Read the model definition and answer for the solid it produces. Units are mm, in the model's axes. Face numbers are marked on the shaded views. A direction names the side the tool comes from. Coordinates: 2 decimals unless noted, no trailing zeros. Loops run counter-clockwise (first coordinate to the right, second up) from the corner with the lowest first, then second, coordinate; pieces in that order, holes last. Notation, with made-up numbers: M 75,5 L 112,5 A24 ccw 112,27 Z; hole C 73,47.25 d5. An arc over 180 degrees is marked long. One line per item, written item: value. Start each with the question number.
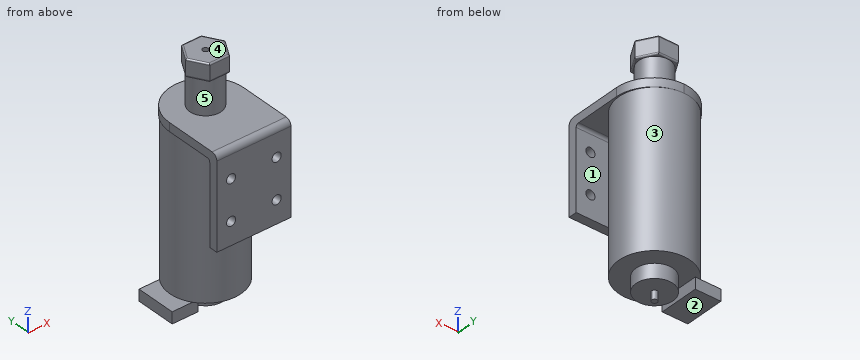
Autodesk Inventor part; units mm, degrees
ref_plane "YZ Plane" through (0, 0, 0) normal (1, 0, 0) x (0, 1, 0)
ref_plane "XZ Plane" through (0, 0, 0) normal (0, 1, 0) x (-1, 0, 0)
ref_plane "XY Plane" through (0, 0, 0) normal (0, 0, 1) x (1, 0, 0)
sketch "Эскиз1" plane through (0, 0, 0) normal (0, 1, 0) x (-1, 0, 0)
  line L0 (0, 0) -> (-26, 0)
  line L1 (0, -32) -> (-26, -32)
  line L2 (-26, -32) -> (0, -32)
  line L3 (0, -32) -> (0, 0)
  line L4 (0, 0) -> (-26, 0)
  line L5 (-26, 0) -> (-26, -32)
extrude "Выдавливание1" add sketch "Эскиз1" along normal blind 3
sketch "Эскиз2" plane through (0, 3, 0) normal (0, 1, 0) x (1, 0, 0)
  line L0 (0, 0) -> (26, 0)
  line L1 (26, 0) -> (26, 33)
  line L2 (0, 0) -> (26, 0)
  line L3 (26, 0) -> (26, 3)
  line L4 (26, 3) -> (0, 3)
  line L5 (0, 3) -> (0, 0)
  dimension "d4" = 3
extrude "Выдавливание2" add sketch "Эскиз2" along normal blind 30
sketch "Эскиз3" plane through (26, 3, -3) normal (0, 0, -1) x (-1, 0, 0)
  line L0 (0, 0) -> (26, 0)
  line L1 (13, 0) -> (13, 5)
  line L2 (13, 5) -> (13, 17.5)
  circle A0 centre (13, 17.5) radius 12.5
  point P0 (26, -3)
  dimension "d7" = 5
  dimension "d8" = 12.5
extrude "Выдавливание3" add sketch "Эскиз3" along normal blind 61.8
sketch "Эскиз4" plane through (13, 20.5, -64.8) normal (0, 0, -1) x (-1, 0, 0)
  circle A0 centre (0, 0) radius 6.5
  circle A1 centre (0, 0) radius 12.5
  point P0 (13, -20.5)
  dimension "d11" = 13
extrude "Выдавливание4" cut sketch "Эскиз4" against normal blind 8
sketch "Эскиз5" plane through (13, 20.5, -64.8) normal (0, 0, -1) x (-1, 0, 0)
  circle A0 centre (0, 0) radius 1
  circle A1 centre (0, 0) radius 6.5
  point P0 (13, -20.5)
  dimension "d14" = 2
extrude "Выдавливание5" cut sketch "Эскиз5" against normal blind 3
sketch "Эскиз6" plane through (13, 20.5, -56.8) normal (0, 0, -1) x (-1, 0, 0)
  circle A0 centre (0, 0) radius 12.5
  line L0 (-12.5, 0) -> (8.5, 0)
  line L1 (8.5, 0) -> (8.5, 7)
  line L2 (8.5, 7) -> (17.5, 7)
  line L3 (17.5, 7) -> (17.5, -7)
  line L4 (17.5, -7) -> (8.5, -7)
  line L5 (8.5, -7) -> (8.5, 0)
  point P0 (13, -20.5)
  dimension "d17" = 21
  dimension "d18" = 7
  dimension "d19" = 9
  dimension "d20" = 14
extrude "Выдавливание6" add sketch "Эскиз6" along normal blind 4 contours A0 L4 L5 L1 L2 | A0 L2 L3 L4
sketch "Эскиз7" plane through (0, 0, 0) normal (0, 0, 1) x (1, 0, 0)
  circle A0 centre (13, 20.5) radius 1
  circle A1 centre (13, 20.5) radius 5.5
  point P0 (0, 0)
  dimension "d23" = 11
extrude "Выдавливание7" add sketch "Эскиз7" along normal blind 12 contours A0 | A1
sketch "Эскиз8" plane through (13, 20.5, 12) normal (0, 0, 1) x (1, 0, 0)
  line L0 (0, 0) -> (0, 6)
  circle A0 centre (0, 0) radius 1
  line L1 (3.4641, 6) -> (6.9282, 0)
  line L2 (6.9282, 0) -> (3.4641, -6)
  line L3 (3.4641, -6) -> (-3.4641, -6)
  line L4 (-3.4641, -6) -> (-6.9282, 0)
  line L5 (-6.9282, 0) -> (-3.4641, 6)
  line L6 (-3.4641, 6) -> (3.4641, 6)
  point P0 (-13, -20.5)
  dimension "d26" = 6
extrude "Выдавливание8" add sketch "Эскиз8" along normal blind 6
fillet "Сопряжение1" radius 0.5 12 edges at (7.8038, 23.5, 12) (13, 26.5, 12) (7.8038, 17.5, 12) (13, 14.5, 12) (18.1962, 17.5, 12) (18.1962, 23.5, 12) (13, 14.5, 18) (18.1962, 17.5, 18) (18.1962, 23.5, 18) (13, 26.5, 18) (7.8038, 23.5, 18) (7.8038, 17.5, 18)
sketch "Эскиз9" plane through (0, 0, 0) normal (0, -1, 0) x (1, 0, 0)
  line L0 (26, 0) -> (26, -33)
  line L1 (0, 0) -> (26, 0)
  line L2 (5, -10) -> (21, -10)
  line L3 (21, -10) -> (21, -24)
  line L4 (21, -24) -> (5, -24)
  line L5 (5, -24) -> (5, -10)
  circle A0 centre (5, -10) radius 1.6
  circle A1 centre (21, -10) radius 1.6
  circle A2 centre (21, -24) radius 1.6
  circle A3 centre (5, -24) radius 1.6
  dimension "d45" = 16
  dimension "d46" = 14
  dimension "d47" = 3.2
  dimension "d48" = 3.2
  dimension "d49" = 3.2
  dimension "d50" = 3.2
extrude "Выдавливание9" cut sketch "Эскиз9" against normal blind 3 contours L5 A0 L2 | L2 A0 L5 | A1 L3 L2 | L2 L3 A1 | A3 L4 L5 | L5 L4 A3 | A2 L4 L3 | L3 L4 A2
fillet "Сопряжение2" radius 2 1 edges at (13, 0, 0)
fillet "Сопряжение3" radius 1 1 edges at (13, 3, -3)
fillet "Сопряжение4" radius 13 2 edges at (0, 33, -1.5) (26, 33, -1.5)
properties part number "motor"
1) Consider line 1 along X through (y, z) = (1, -10); line 2 along Z through (x, y) = (5, 1.3); line 3 along Z through (x, y) = (5, 1). Determine where each line is inside the solid, lowest interval first.
2) Flat-ended cylindrical pins translate along their axes: pin 1 (2 mm diameter, centred on y = 18, z = -58, fed in from +X); pin 2 (2 mm diameter, centred on x = 15, y = 18, fed in from -Z); pin 3 (1 mm diameter, centred on y = 27, z = -36.5, fed in from -X). Find the tip coordinate at first contact, or state that the pin passes through.
3) Section B-B (z = -59) is taken. Determine the outline of the cut face in (x, y), then the cut area to 3 significant figures.
4) Section A-A (z = -10) is taken. Determine the outline of the cut face in (x, y).
5) Section C-C (x = 21) is taken. Determine the outline of the cut face in (y, z).
6) Section D-D (y = 10) is taken. Determine the outline of the cut face in (x, z).
7) For a pull along Z with two mould halves and no side action, classify the marked faces 1, 2 and 3 as released by +Z, released by -Z, zero draft, split by the parting line, or undercut.
8) A tool of negligible diameter and unlimited length cuts with its end or side. For the marked faces 4 and 5, from which of +Z, -Z, +X, -X, +Y, -Y can it reach the whole face along a straight path? Write none if from no direction.
Results found:
1. line 1: x = 0 to 3.4, 6.6 to 19.4, 22.6 to 26
1. line 2: z = -32 to -25.6, -22.4 to -11.6, -8.4 to -0.13
1. line 3: z = -32 to -25.6, -22.4 to -11.6, -8.4 to -0.27
2. pin 1: stops at x = 19.32
2. pin 2: stops at z = -61.8
2. pin 3: stops at x = 2.03
3. outline: M -4.5,13.5 L 4.5,13.5 L 4.5,27.5 L -4.5,27.5 Z; C 13,20.5 d13
3. area: 259 mm²
4. outline: M 0,0 L 3.4,0 L 3.4,3 L 0,3 Z; C 13,20.5 d25; M 6.6,0 L 19.4,0 L 19.4,3 L 6.6,3 Z; M 22.6,0 L 26,0 L 26,3 L 22.6,3 Z
5. outline: M 0,-32 L 3,-32 L 3,-25.6 L 0,-25.6 Z; M 0,-22.4 L 3,-22.4 L 3,-11.6 L 0,-11.6 Z; M 0,-8.4 L 3,-8.4 L 3,-4 A1 cw 4,-3 L 10.9,-3 L 10.9,-56.8 L 30.1,-56.8 L 30.1,-3 L 30.25,-3 L 30.25,0 L 2,0 A2 ccw 0,-2 Z
6. outline: M 0,-3 L 6.22,-3 L 6.22,-56.8 L 19.78,-56.8 L 19.78,-3 L 26,-3 L 26,0 L 0,0 Z
7. face 1: zero draft
7. face 2: released by -Z
7. face 3: undercut
8. face 4: +Z, +X, -X, +Y, -Y
8. face 5: none
